Design review of the part shown in the three views and the two pictorial views. Dimensions are in mm from the part's minimum x, y and z. Give positions to 0.01 mm unless a question says otherwise; leave off trailing zeros. Order: outer loops, then holes, each group sorted by start corner. A loop starts at its lowest first (then second) coordinate and runs counter-clockwise, first axis right, second up.
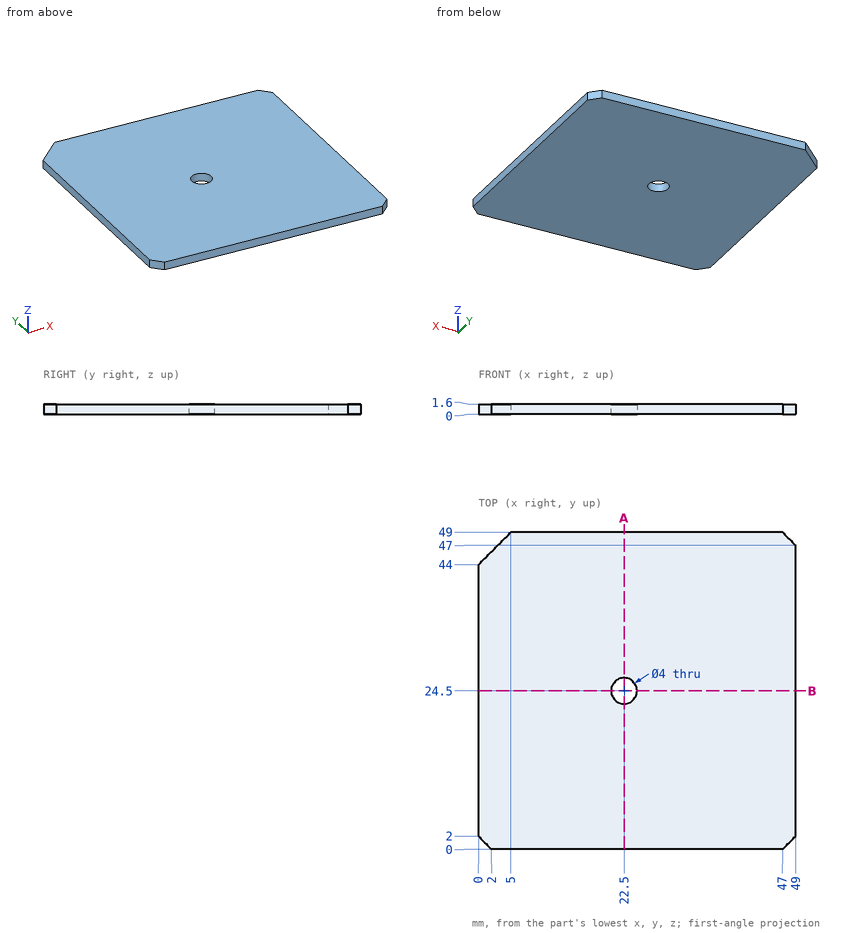
1) To check wall thickness, follow line 1 (Y direction, x = 22.5, z = 1.15); line 2 (Y direction, x = 23, z = 0.6); line 3 (X direction, y = 46, z = 0.7). State the ranges of each line that lie inside material, in increasing order.
Answer sheet:
line 1: y = 0 to 22.5, 26.5 to 49
line 2: y = 0 to 22.56, 26.44 to 49
line 3: x = 2 to 49
2) We need section B-B on y = 24.5. Give the boundary of the cut face in (x, z).
Answer sheet:
outline: (0, 0) - (20.5, 0) - (20.5, 1.6) - (0, 1.6) - close; (24.5, 0) - (49, 0) - (49, 1.6) - (24.5, 1.6) - close
3) We need section A-A on x = 22.5. Give the boundary of the cut face in (y, z).
Answer sheet:
outline: (0, 0) - (22.5, 0) - (22.5, 1.6) - (0, 1.6) - close; (26.5, 0) - (49, 0) - (49, 1.6) - (26.5, 1.6) - close
4) Clearance check with a flat-ended pin moving along its axis: pin 1 (2 mm diameter, centred on x = 28.5, y = 30.5, fed in from -Z). State where the tip first meets the part, or that it passes through.
Answer sheet:
pin 1: stops at z = 0
